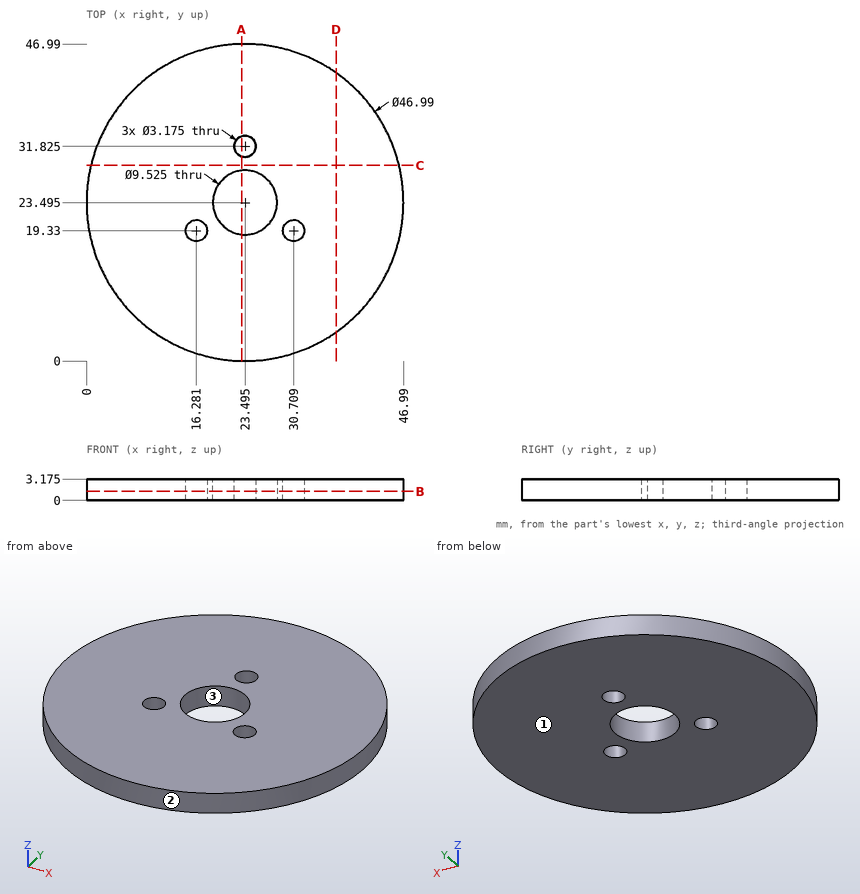
Study the drawing (mm; zero at the part's minimum x, y, z) and answer. Round coordinates to 2 decimals unless told otherwise and drop trailing zeros. Loops run counter-clockwise (first coordinate to the right, second up) from the corner with the lowest first, then second, coordinate; pieces in that order, holes last. Notation, with made-up numbers: (4.25, -22) -> (63.25, -22) arc R35 ccw to (63.25, 14) -> close; hole circle Ø11 at (13.5, 89.25). An arc over 180 degrees is marked (long way). Use one line per item in the form item = value.
1. The part is cut by section C-C on y = 29. Determine the outline of the cut face in (x, z) (1 decimal).
Answer key:
outline = (0.7, 0) -> (46.3, 0) -> (46.3, 3.2) -> (0.7, 3.2) -> close
2. A flat-ended cylindrical pin translates along its axis: pin 1 Ø5 at (x, y) = (23.5, 31.82) entering from +Z (1 decimal). Find the tip coordinate at first contact, or state that the pin passes through.
Answer key:
pin_1 = 3.2
3. Find the intervals of material crossed by probe 1 along Y at (x, z) = (23.5, 1.15); probe 2 along X at (y, z) = (22.5, 0.2); probe 3 along Y at (x, z) = (30, 1.3), in increasing order. Write a range as [from, to].
Answer key:
probe_1 = [0, 18.73], [28.26, 30.24], [33.41, 46.99]
probe_2 = [0.02, 18.84], [28.15, 46.97]
probe_3 = [0.92, 17.91], [20.75, 46.07]
4. For a pull along Y with two mould halves and no side action, classify the marked faces 1, 2 and 3 as released by +Y, released by -Y, zero draft, split by the parting line, or undercut.
Answer key:
face_1 = zero draft
face_2 = split by the parting line
face_3 = undercut
5. The part is cut by section B-B on z = 1.35. Determine the outline of the cut face in (x, y) (1 decimal).
Answer key:
outline = circle Ø47 at (23.5, 23.5); hole circle Ø3.2 at (16.3, 19.3); hole circle Ø9.5 at (23.5, 23.5); hole circle Ø3.2 at (23.5, 31.8); hole circle Ø3.2 at (30.7, 19.3)
6. The part is cut by section A-A on x = 23. Determine the outline of the cut face in (y, z) (1 decimal).
Answer key:
outline = (0, 0) -> (18.8, 0) -> (18.8, 3.2) -> (0, 3.2) -> close; (28.2, 0) -> (30.3, 0) -> (30.3, 3.2) -> (28.2, 3.2) -> close; (33.3, 0) -> (47, 0) -> (47, 3.2) -> (33.3, 3.2) -> close
7. The part is cut by section D-D on x = 37. Determine the outline of the cut face in (y, z) (1 decimal).
Answer key:
outline = (4.3, 0) -> (42.7, 0) -> (42.7, 3.2) -> (4.3, 3.2) -> close
